Could you check a few things on this model? Use its own coordinates, in mm. Give positions to 0.01 mm unless a question says otherwise; leave off trailing zeros. Loops run counter-clockwise (first coordinate to the right, second up) from the corner with the lowest first, then second, coordinate; pieces in that order, holes last. Notation, with made-up numbers: (-13, 21) -> (25, 21) arc R15 ccw to (25, 35) -> close; hole circle Ø1 at (30.5, -13.5). An arc over 180 degrees is marked (long way). Write item = value, one per line. Start each with the question number.
1) I want a section at A-A (x = 52.5). List the corners of the cut face in (y, z) for me, and give its area (3 significant figures).
2) I need wall thicknesses on probe 1 along Z at (x, y) = (65.5, -0.1); probe 2 along Z at (x, y) = (-20, -0.45); probe 3 along Y at (x, z) = (39.5, 12.75). Which ranges of each line are inside material? Lowest first, please. Write a range as from..to.
3) I want a section at C-C (z = 13.75). List the corners of the cut face in (x, y) for me.
4) I'm going to push flat-ended pins straight in: pin 1 Ø2 at (x, z) = (72, 14.5) entering from +Y; pin 2 Ø1.5 at (x, y) = (105.5, -1) entering from -Z. Where does each tip first touch, or does it pass through?
5) I want a section at B-B (y = 1.25). List the corners of the cut face in (x, z) for me, and give its area (3 significant figures).
from build123d import *

# Parameters (mm, degrees)
SKETCH1_W           = 175.4666
SKETCH1_H           = 3
SKETCH3_R           = 3
BOSS_EXTRUDE1_DEPTH = 10
SKETCH7_R           = 3
BOSS_EXTRUDE5_DEPTH = 3


with BuildPart() as part:
    # Sketch1 → Revolve2 (revolve)
    with BuildSketch(Plane(origin=(0, 0, 0), x_dir=(1, 0, 0), z_dir=(0, 1, 0)), mode=Mode.PRIVATE) as revolve2_sk:
        with Locations((46.032622124, -14.621103214)):
            Rectangle(SKETCH1_W, SKETCH1_H)
    revolve(revolve2_sk.sketch.rotate(Axis((133.765922124, 0, 13.121103214), (-1, 0, 0)), 180), axis=Axis((133.765922124, 0, 13.121103214), (-1, 0, 0)))

    # Sketch3 → Boss-Extrude1 (add)
    with BuildSketch(Plane.ZY.offset(41.700677876)):
        with Locations(Location((13.121103214, 0, 0), (0, 0, 180))):
            Circle(SKETCH3_R)
    extrude(amount=BOSS_EXTRUDE1_DEPTH)

    # Sketch7 → Boss-Extrude5 (add)
    with BuildSketch(Plane.ZY.offset(51.700677876)):
        with Locations(Location((13.121103214, 0, 0), (0, 0, 180))):
            Circle(SKETCH7_R)
    extrude(amount=BOSS_EXTRUDE5_DEPTH)


solid = part.part
Answer list:
q1.outline = circle Ø6 at (0, 13.12)
q1.area = 28.3 mm^2
q2.probe_1 = 10.12..16.12
q2.probe_2 = 10.16..16.09
q2.probe_3 = -2.98..2.98
q3.outline = (-54.7, -2.93) -> (133.77, -2.93) -> (133.77, 2.93) -> (-54.7, 2.93) -> close
q4.pin_1 = 2.98
q4.pin_2 = 10.13
q5.outline = (-54.7, 10.39) -> (133.77, 10.39) -> (133.77, 15.85) -> (-54.7, 15.85) -> close
q5.area = 1,030 mm^2
